```python
from build123d import *

# Parameters (mm, degrees)
SKETCH1_W           = 101.6
SKETCH1_H           = 50.8
BOSS_EXTRUDE1_DEPTH = 1524
SKETCH2_R           = 3.4925
CUT_EXTRUDE1_DEPTH  = 50.8
SKETCH3_R           = 15.875
CUT_EXTRUDE2_DEPTH  = 101.6


with BuildPart() as part:
    # Sketch1 → Boss-Extrude1 (new body)
    with BuildSketch(Plane.XY):
        Rectangle(SKETCH1_W, SKETCH1_H)
    extrude(amount=BOSS_EXTRUDE1_DEPTH)

    # Sketch2 → Cut-Extrude1 (cut)
    with BuildSketch(Plane(origin=(0, 25.4, 0), x_dir=(1, 0, 0), z_dir=(0, 1, 0))):
        with Locations(Location((-25.4, -1447.8, 0), (0, 0, 270))):
            Circle(SKETCH2_R)
        with Locations(Location((25.4, -1447.8, 0), (0, 0, 270))):
            Circle(SKETCH2_R)
        with Locations(Location((25.4, -1498.6, 0), (0, 0, 270))):
            Circle(SKETCH2_R)
        with Locations(Location((-25.4, -1498.6, 0), (0, 0, 270))):
            Circle(SKETCH2_R)
    extrude(amount=-CUT_EXTRUDE1_DEPTH, mode=Mode.SUBTRACT)

    # Sketch3 → Cut-Extrude2 (cut)
    with BuildSketch(Plane(origin=(50.8, 0, 0), x_dir=(0, 0, -1), z_dir=(1, 0, 0))):
        with Locations((-101.6, 0)):
            Circle(SKETCH3_R)
    extrude(amount=-CUT_EXTRUDE2_DEPTH, mode=Mode.SUBTRACT)


solid = part.part
```
Input: part model. Units: mm. Frame: model coordinates. Coordinates: 2 decimals unless noted, no trailing zeros. Write each loop counter-clockwise with the first axis right and the second up, starting at its lowest first coordinate (ties: lowest second). Pieces come first, ordered by that corner, then holes.
1) Section A-A on y = 0. Output: boundary loops of the cut face in (x, z) (1 decimal).
2) Section B-B on z = 101.6. Output: boundary loops of the cut face in (x, y) (3 decimals).
3) Material intervals for line 1 along X through (y, z) = (2, 1498); line 2 along X through (y, z) = (-7, 1498.6); line 3 along Z through (x, y) = (25, -11), sorted ascending.
4) Mould query, pull axis Z, two halves, no side actions, for faces 1 (the flat face through (50.8, 0, 751)), 2 (the flat face through (-1, 0, 0)), 3 (the cylindrical face through (0.71, 0.7, 117.46)). Classes: pulls with the +Z half, pulls with the -Z half, needs draft (parallel to the pull), parting line crosses it, or undercut.
Check result:
1. outline: (-50.8, 0) - (50.8, 0) - (50.8, 85.7) - (-50.8, 85.7) - close; (-50.8, 117.5) - (50.8, 117.5) - (50.8, 1524) - (-50.8, 1524) - close; hole circle Ø7 at (-25.4, 1447.8); hole circle Ø7 at (-25.4, 1498.6); hole circle Ø7 at (25.4, 1447.8); hole circle Ø7 at (25.4, 1498.6)
2. outline: (-50.8, -25.4) - (50.8, -25.4) - (50.8, -15.875) - (-50.8, -15.875) - close; (-50.8, 15.875) - (50.8, 15.875) - (50.8, 25.4) - (-50.8, 25.4) - close
3. line 1: x = -50.8 to -28.84, -21.96 to 21.96, 28.84 to 50.8
3. line 2: x = -50.8 to -28.89, -21.91 to 21.91, 28.89 to 50.8
3. line 3: z = 0 to 90.15, 113.05 to 1444.33, 1451.27 to 1495.13, 1502.07 to 1524
4. face 1: needs draft
4. face 2: pulls with the -Z half
4. face 3: undercut
